Verification items for the finished model (mm, model axes). Face numbers are marked on the shaded views. A direction names the side the tool comes from. Round coordinates to 2 decimals unless told otherwise and drop trailing zeros. Order: outer loops, then holes, each group sorted by start corner. A loop starts at its lowest first (then second) coordinate and runs counter-clockwise, first axis right, second up.
```python
from build123d import *

# Parameters (mm, degrees)
F1_DEPTH  = 140
F2_W      = 12
F2_H      = 140
F3_DEPTH  = 206
F4_W      = 140
F4_H      = 12
F5_DEPTH  = 188
F6_W      = 12
F6_H      = 140
F7_DEPTH  = 200
F8_W      = 140
F8_H      = 12
F9_DEPTH  = 188
F10_R     = 9.5
F11_DEPTH = 200
F13_DEPTH = 200


with BuildPart() as f1:
    # F0 (on Front) → F1 (new body)
    with BuildSketch(Plane.XZ):
        Polygon((12, 6), (12, 0), (200, 0), (200, 12), (0, 12), (0, 6), align=None)
    extrude(amount=-F1_DEPTH)

    # F2 (on face) → F3 (join)
    with BuildSketch(Plane(origin=(0, 0, 6), x_dir=(1, 0, 0), z_dir=(0, 0, -1))):
        with Locations((6, -70)):
            Rectangle(F2_W, F2_H)
    extrude(amount=F3_DEPTH)

    # F4 (on face) → F5 (join)
    with BuildSketch(Plane.YZ.offset(12)):
        with Locations((70, -194)):
            Rectangle(F4_W, F4_H)
    extrude(amount=F5_DEPTH)

    # F6 (on face) → F7 (join)
    with BuildSketch(Plane(origin=(0, 0, -200), x_dir=(1, 0, 0), z_dir=(0, 0, -1))):
        with Locations((194, -70)):
            Rectangle(F6_W, F6_H)
    extrude(amount=F7_DEPTH)

    # F8 (on face) → F9 (join)
    with BuildSketch(Plane(origin=(188, 0, 0), x_dir=(0, -1, 0), z_dir=(-1, 0, 0))):
        with Locations((-70, -394)):
            Rectangle(F8_W, F8_H)
    extrude(amount=F9_DEPTH)

    # F10 (on face) → F11 (join)
    with BuildSketch(Plane.XY.offset(-388)):
        with Locations((30, 30)):
            Circle(F10_R)
        with Locations((30, 110)):
            Circle(F10_R)
    extrude(amount=F11_DEPTH)

    # F12 (on face) → F13 (join)
    with BuildSketch(Plane.XY.offset(-188)):
        with BuildLine():
            ThreePointArc((179.5, 110), (176.717514, 116.717514), (170, 119.5))
            Line((170, 119.5), (170, 110))
            Line((170, 110), (179.5, 110))
        make_face()
        with BuildLine():
            Line((170, 110), (170, 119.5))
            ThreePointArc((170, 119.5), (163.282486, 103.282486), (179.5, 110))
            Line((179.5, 110), (170, 110))
        make_face()
        with BuildLine():
            ThreePointArc((170, 20.5), (176.717514, 23.282486), (179.5, 30))
            Line((179.5, 30), (170, 30))
            Line((170, 30), (170, 20.5))
        make_face()
        with BuildLine():
            Line((170, 30), (179.5, 30))
            ThreePointArc((179.5, 30), (163.282486, 36.717514), (170, 20.5))
            Line((170, 20.5), (170, 30))
        make_face()
    extrude(amount=F13_DEPTH)


solid = f1.part
```
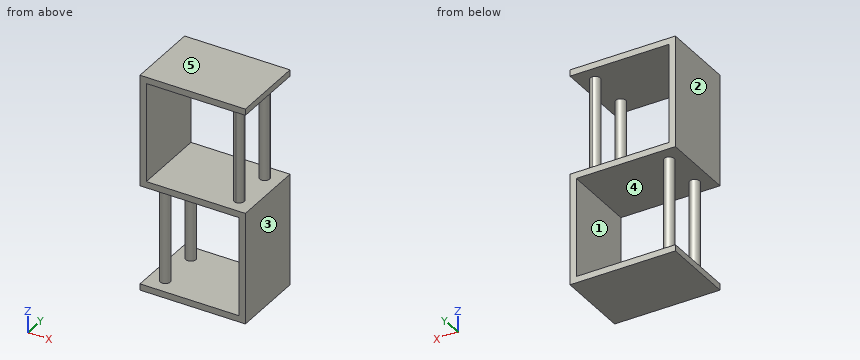
1) Sectioned sample at C-C on y = 66.5. Record the cut outline in (x, z), then the cut area to 3 significant figures.
2) Sectioned sample at A-A on z = -89.5. Record the cut outline in (x, y), then the cut area to 3 significant figures.
3) Scan lines: probe 1 along Z at (x, y) = (125.5, 109); probe 2 along Z at (x, y) = (27, 38); probe 3 along X at (y, z) = (111, -185.5). Record each from-to range of solid material in increasing order.
4) Sectioned sample at B-B on x = 16. Record the cut outline in (y, z), then the cut area to 3 significant figures.
5) Go/stop test with flat-tipped pins: pin 1 Ø5 at (x, z) = (32, -294.5) entering from -Y; pin 2 Ø1 at (x, z) = (163, -177.5) entering from -Y; pin 3 Ø2 at (y, z) = (15.5, -94) entering from +X. Record where each tip stops, or that it passes through.
6) Draft check along X on the marked faces 3, 4 and 5. Enter one of: released by +X, released by -X, zero draft, split by the parting line, or undercut.
7) Tool access check on the marked faces 1 and 2. Record the directions out of +Z, -Z, +X, -X, +Y, -Y that give a thin tool (end or side, any length) a straight path to the whole face; none if there is none.
Returned:
1. outline: (0, -400) - (200, -400) - (200, -188) - (12, -188) - (12, 0) - (200, 0) - (200, 12) - (0, 12) - (0, -200) - (188, -200) - (188, -388) - (0, -388) - close
1. area: 11,700 mm2
2. outline: (0, 0) - (12, 0) - (12, 140) - (0, 140) - close; (170, 20.5) arc R9.5 ccw to (179.5, 30) arc R9.5 ccw (long way) to start; (170, 119.5) arc R9.5 ccw (long way) to (179.5, 110) arc R9.5 ccw to start
2. area: 2,250 mm2
3. probe 1: z = -400 to -388, -200 to -188, 0 to 12
3. probe 2: z = -400 to -188, 0 to 12
3. probe 3: x = 0 to 12, 160.55 to 179.45
4. outline: (0, -400) - (140, -400) - (140, -388) - (0, -388) - close; (0, -200) - (140, -200) - (140, -188) - (0, -188) - close; (0, 0) - (140, 0) - (140, 12) - (0, 12) - close
4. area: 5,040 mm2
5. pin 1: stops at y = 20.5
5. pin 2: stops at y = 23.07
5. pin 3: stops at x = 12
6. face 3: released by +X
6. face 4: undercut
6. face 5: zero draft
7. face 1: +Y, -Y
7. face 2: +Z, -Z, -X, +Y, -Y
